Check sheet for the modelled part. Datum: model origin and axes. Units: mm. A direction names the side the tool comes from. Round coordinates to 2 decimals unless told otherwise and drop trailing zeros. Order: outer loops, then holes, each group sorted by start corner. A loop starts at its lowest first (then second) coordinate and runs counter-clockwise, first axis right, second up. Notation, with made-up numbers: (83.25, -33) -> (88.25, -33) arc R25 cw to (88.25, -21) -> close; hole circle Ø7 at (78.5, 11). An arc over 180 degrees is marked (long way). Answer in a Markdown table with one row per item.
Autodesk Inventor part; units mm, degrees
ref_plane "YZ Plane" through (0, 0, 0) normal (1, 0, 0) x (0, 1, 0)
ref_plane "XZ Plane" through (0, 0, 0) normal (0, 1, 0) x (-1, 0, 0)
ref_plane "XY Plane" through (0, 0, 0) normal (0, 0, 1) x (1, 0, 0)
sketch "Sketch1" plane through (0, 0, 0) normal (1, 0, 0) x (0, 1, 0)
  line L0 (6.1324, -14.2794) -> (-5.8676, -14.2794)
  line L1 (-5.8676, -14.2794) -> (-5.8676, -43.2794)
  line L2 (-5.8676, -43.2794) -> (6.1324, -43.2794)
  line L3 (6.1324, -43.2794) -> (6.1324, -14.2794)
  point P0 (0, 0)
  dimension "d0" = 12
  dimension "d1" = 29
extrude "Extrusion1" add sketch "Sketch1" along normal blind 1.8
sketch "Sketch2" plane through (1.8, 0, 0) normal (1, 0, 0) x (0, 0, -1)
  circle A0 centre (38.2794, 0.1324) radius 3.5
  line L0 (43.2794, -5.8676) -> (43.2794, 6.1324)
  line L1 (14.2794, -5.8676) -> (43.2794, -5.8676)
  point P0 (0, 0)
  dimension "d4" = 7
  dimension "d5" = 5
  dimension "d6" = 6
extrude "Extrusion2" cut sketch "Sketch2" against normal blind 0.8
sketch "Sketch3" plane through (1.8, 0, 0) normal (1, 0, 0) x (0, 0, -1)
  line L0 (14.2794, 6.1324) -> (14.2794, -5.8676)
  line L1 (43.2794, -5.8676) -> (43.2794, 6.1324)
  line L2 (14.2794, 6.1324) -> (43.2794, 6.1324)
  line L3 (43.2794, 6.1324) -> (43.2794, -5.8676)
  line L4 (43.2794, -5.8676) -> (14.2794, -5.8676)
  line L5 (14.2794, -5.8676) -> (14.2794, 6.1324)
  circle A0 centre (38.2794, 0.1324) radius 3.5
  circle A1 centre (38.2794, 0.1324) radius 3.5
  point P0 (0, 0)
  point P1 (43.2794, 6.1324)
  point P2 (14.2794, -5.8676)
extrude "Extrusion3" add sketch "Sketch3" along normal blind 2.5
sketch "Sketch4" plane through (4.3, 0, 0) normal (1, 0, 0) x (0, 0, -1)
  circle A0 centre (38.2794, 0.1324) radius 3.5
  line L0 (36.7494, 3.2802) -> (22.3405, 1.8824)
  line L1 (36.7494, -3.0155) -> (22.3405, -1.6176)
  arc A1 (22.3405, 1.8824) -> (22.3405, -1.6176) centre (24.7889, 0.1324) ccw
  line L2 (43.2794, 6.1324) -> (14.2794, 6.1324)
  point P0 (0, 0)
  point P1 (21.7794, 0.1324)
  dimension "d15" = 1.53
  dimension "d16" = 1.53
  dimension "d17" = 16.5
  dimension "d18" = 3.5
  dimension "d19" = 6
extrude "Extrusion4" cut sketch "Sketch4" against normal blind 2.5 contours A0 L1 A1 L0
sketch "Sketch5" plane through (0, 0, 0) normal (-1, 0, 0) x (0, 0, 1)
  circle A0 centre (-38.2794, 0.1324) radius 3.5
  circle A1 centre (-38.2794, 0.1324) radius 1.25
  point P0 (0, 0)
  dimension "d22" = 2.5
extrude "Extrusion5" cut sketch "Sketch5" against normal blind 2.5 contours A1
sketch "Sketch6" plane through (4.3, 0, 0) normal (1, 0, 0) x (0, 0, -1)
  line L0 (43.2794, 6.1324) -> (14.2794, 6.1324)
  line L1 (14.2794, -5.8676) -> (43.2794, -5.8676)
  line L2 (14.2794, 6.1324) -> (17.2794, 6.1324)
  line L3 (17.2794, 6.1324) -> (17.2794, -5.8676)
  line L4 (17.2794, -5.8676) -> (14.2794, -5.8676)
  line L5 (14.2794, -5.8676) -> (14.2794, 6.1324)
  point P0 (0, 0)
  point P1 (14.2794, -5.8676)
  point P2 (17.2794, 6.1324)
  dimension "d25" = 3
extrude "Extrusion6" add sketch "Sketch6" along normal blind 35
sketch "Sketch7" plane through (0, -5.8676, -14.2794) normal (0, 0, 1) x (1, 0, 0)
  circle A0 centre (28.925, 6) radius 1.5
  line L0 (39.3, 12) -> (39.3, 0)
  line L1 (0, 12) -> (39.3, 12)
  line L2 (0, 12) -> (0, 0)
  point P0 (0, 5.8676)
  dimension "d28" = 3
  dimension "d30" = 6
  dimension "d38" = 28.925
extrude "Extrusion7" cut sketch "Sketch7" against normal blind 40
sketch "Sketch8" plane through (1.8, 0, 0) normal (1, 0, 0) x (0, 0, -1)
  circle A0 centre (25.7794, 0.1324) radius 1
  circle A1 centre (38.2794, 0.1324) radius 1.25
  point P0 (0, 0)
  dimension "d33" = 2
  dimension "d34" = 12.5
  dimension "d35" = 0
extrude "Extrusion8" cut sketch "Sketch8" against normal blind 10 contours A0
properties part number "18_2"
(1) Section check C-C on y = 5.5. Record the boundary of the cut face in (x, z), plus the area to 3 significant figures.
Solutions:
| item | result |
|---|---|
| outline | (0, -43.28) -> (4.3, -43.28) -> (4.3, -17.28) -> (39.3, -17.28) -> (39.3, -14.28) -> (0, -14.28) -> close |
| area | 230 mm^2 |
(2) Section check D-D on z = -31.75. Record the boundary of the cut face in (x, y), plus the area to 3 significant figures.
Solutions:
| item | result |
|---|---|
| outline | (0, -5.87) -> (4.3, -5.87) -> (4.3, -2.53) -> (1.8, -2.53) -> (1.8, 2.8) -> (4.3, 2.8) -> (4.3, 6.13) -> (0, 6.13) -> close |
| area | 38.3 mm^2 |
(3) Tool access check on faces 1 (the flat face through (22, 0, -17.279)), 2 (the cylindrical face through (30.356, 0.583, -15.758)), 3 (the flat face through (3.068, -2.326, -29.646)). Record the directions out of +Z, -Z, +X, -X, +Y, -Y that give a thin tool (end or side, any length) a straight path to the whole face; none if there is none.
Solutions:
| item | result |
|---|---|
| face 1 | -Z, +X, +Y, -Y |
| face 2 | +Z, -Z |
| face 3 | +X |
(4) Scan lines: probe 1 along Y at (x, z) = (2, -38.5); probe 2 along Z at (x, y) = (38, 3.75); probe 3 along X at (y, z) = (-2.75, -23.75). Record each from-to range of solid material in increasing order. Write a range as from..to.
Solutions:
| item | result |
|---|---|
| probe 1 | -5.87..-3.36, 3.63..6.13 |
| probe 2 | -17.28..-14.28 |
| probe 3 | 0..4.3 |
(5) Depth check by flat-ended pin: pin 1 Ø3 at (y, z) = (-4, -23) entering from +X; pin 2 Ø3 at (y, z) = (0.13, -25.78) entering from +X; pin 3 Ø3 at (x, y) = (29.5, 1.5) entering from -Z. Enter the tip coordinate at first touch or a pass-through.
Solutions:
| item | result |
|---|---|
| pin 1 | x = 4.3 |
| pin 2 | x = 1.8 |
| pin 3 | z = -17.28 |
(6) Section check A-A on x = 29. Record the boundary of the cut face in (y, z).
Solutions:
| item | result |
|---|---|
| outline | (-5.87, -17.28) -> (-1.37, -17.28) -> (-1.37, -14.28) -> (-5.87, -14.28) -> close; (1.63, -17.28) -> (6.13, -17.28) -> (6.13, -14.28) -> (1.63, -14.28) -> close |
(7) Draft check along Y on faces 4 (the flat face through (3.07, 2.59, -29.65)), 5 (the flat face through (0, 0, -29)), 6 (the flat face through (11, -5.868, -17)). Enter one of: pulls with the +Y half, pulls with the -Y half, needs draft (parallel to the pull), parting line crosses it, or undercut.
Solutions:
| item | result |
|---|---|
| face 4 | undercut |
| face 5 | needs draft |
| face 6 | pulls with the -Y half |
(8) Section check B-B on z = -38.5. Record the boundary of the cut face in (x, y).
Solutions:
| item | result |
|---|---|
| outline | (0, -5.87) -> (4.3, -5.87) -> (4.3, -3.36) -> (1, -3.36) -> (1, -1.1) -> (0, -1.1) -> close; (0, 1.36) -> (1, 1.36) -> (1, 3.63) -> (4.3, 3.63) -> (4.3, 6.13) -> (0, 6.13) -> close |
